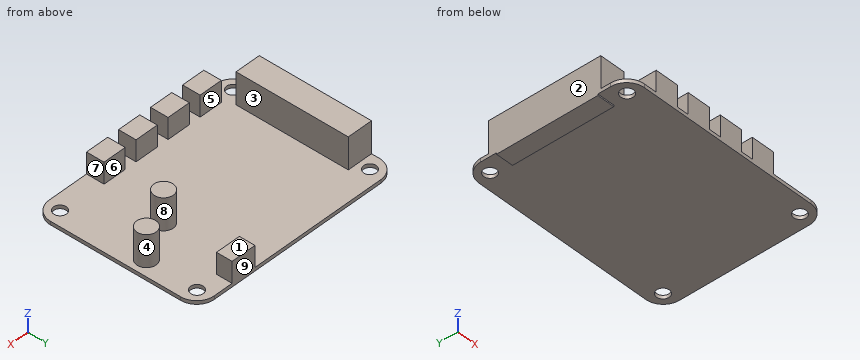
```python
from build123d import *

# Parameters (mm, degrees)
SKETCH_2_R      = 1.8
EXTRUDE_1_DEPTH = 1
SKETCH_4_W      = 7.237291628
SKETCH_4_H      = 31.958994792
EXTRUDE_2_DEPTH = 9
SKETCH_5_W      = 6.609648953
SKETCH_5_H      = 4.992409467
SKETCH_5_W_2    = 7.131463344
SKETCH_5_H_2    = 4.436954379
EXTRUDE_3_DEPTH = 6
SKETCH_6_R      = 2.75
EXTRUDE_4_DEPTH = 9
SKETCH_7_W      = 5
SKETCH_7_H      = 28.854406725
EXTRUDE_5_DEPTH = 0.4


with BuildPart() as part:
    # 草图2 → 凸台-拉伸1 (new body)
    with BuildSketch(Plane.XY):
        with BuildLine():
            Line((-26, 23.5), (26, 23.5))
            ThreePointArc((26, 23.5), (29.535533906, 22.035533906), (31, 18.5))
            Line((31, 18.5), (31, -18.5))
            ThreePointArc((31, -18.5), (29.535533906, -22.035533906), (26, -23.5))
            Line((26, -23.5), (-26, -23.5))
            ThreePointArc((-26, -23.5), (-29.535533906, -22.035533906), (-31, -18.5))
            Line((-31, -18.5), (-31, 18.5))
            ThreePointArc((-31, 18.5), (-29.535533906, 22.035533906), (-26, 23.5))
        make_face()
        with Locations((27, 19.5)):
            Circle(SKETCH_2_R, mode=Mode.SUBTRACT)
        with Locations(Location((-27, 19.5, 0), (0, 0, 180))):
            Circle(SKETCH_2_R, mode=Mode.SUBTRACT)
        with Locations(Location((27, -19.5, 0), (0, 0, 180))):
            Circle(SKETCH_2_R, mode=Mode.SUBTRACT)
        with Locations((-27, -19.5)):
            Circle(SKETCH_2_R, mode=Mode.SUBTRACT)
    extrude(amount=EXTRUDE_1_DEPTH)

    # 草图4 → 凸台-拉伸2 (add)
    with BuildSketch(Plane.XY.offset(1)):
        with Locations((-27.381354186, 0.304371379)):
            Rectangle(SKETCH_4_W, SKETCH_4_H)
    extrude(amount=EXTRUDE_2_DEPTH)

    # 草图5 → 凸台-拉伸3 (add)
    with BuildSketch(Plane.XY.offset(1)):
        with Locations((-18.965120236, -21.003795266)):
            Rectangle(SKETCH_5_W, SKETCH_5_H)
        with Locations((-8.96367774, -21.003795266)):
            Rectangle(SKETCH_5_W, SKETCH_5_H)
        with Locations((1.037764754, -21.003795266)):
            Rectangle(SKETCH_5_W, SKETCH_5_H)
        with Locations((11.039207249, -21.003795266)):
            Rectangle(SKETCH_5_W, SKETCH_5_H)
        with Locations((16.866134615, 21.281522811)):
            Rectangle(SKETCH_5_W_2, SKETCH_5_H_2)
    extrude(amount=EXTRUDE_3_DEPTH)

    # 草图6 → 凸台-拉伸4 (add)
    with BuildSketch(Plane.XY.offset(1)):
        with Locations((26.719458911, 4.848201251)):
            Circle(SKETCH_6_R)
        with Locations((15.293444682, -0.687190124)):
            Circle(SKETCH_6_R)
    extrude(amount=EXTRUDE_4_DEPTH)

    # 草图7 → 凸台-拉伸5 (add)
    with BuildSketch(Plane(origin=(0, 0, 0), x_dir=(-1, 0, 0), z_dir=(0, 0, -1))):
        with Locations((28.5, -0.417423606)):
            Rectangle(SKETCH_7_W, SKETCH_7_H)
    extrude(amount=EXTRUDE_5_DEPTH)


solid = part.part
```
Input: part model. Units: mm. Frame: model coordinates. Face numbers are marked on the shaded views. A direction names the side the tool comes from. Give positions to 0.01 mm unless a question says otherwise; leave off trailing zeros. Write each loop counter-clockwise with the first axis right and the second up, starting at its lowest first coordinate (ties: lowest second). Pieces come first, ordered by that corner, then holes. Notation, with made-up numbers: (-28.75, 62) - (-9.75, 62) arc R19 cw to (-9.75, 82) - close; hole circle Ø11 at (43.25, -31). An arc over 180 degrees is marked (long way). Write item = value, one per line. Start each with the question number.
1) Cut plane D-D (x = -27). Return loops of the section in (y, z), and give its area (3 significant figures).
2) Material intervals for L1, parallel to X at y = -21.5, z = 6.5; L2, parallel to Y at x = -27, z = 0.7; L3, parallel to Y at x = 14, z = 2.5, sorted ascending. Write a range as [from, to].
3) Reachability of the marked faces 5, 6, 7, 8 and 9 from +Z, -Z, +X, -X, +Y, -Y: full face, straight path, thin tool, end or side. Return the list, or none.
4) Cut plane C-C (z = 2). Return loops of the section in (x, y), and give its area (3 significant figures).
5) Cut plane A-A (x = -18.5). Return loops of the section in (y, z), and give its area (3 significant figures).
6) Pin query (flat end, axial travel): pin 1 (5 mm diameter, centred on x = -10.5, z = 4, fed in from +Y); pin 2 (3 mm diameter, centred on x = 27, y = 19.5, fed in from +Z); pin 3 (1 mm diameter, centred on x = -8, y = 12.5, fed in from -Z); pin 4 (1.8 mm diameter, centred on x = 18, z = 3, fed in from -Y). Return the tip coordinate at first contact, or that it passes through.
7) Cut plane B-B (y = -19.5). Return loops of the section in (x, z), and give its area (3 significant figures).
8) Draft query along X for the marked faces 1, 2, 3 and 4. Return one class per face: pulls with the +X half, pulls with the -X half, needs draft (parallel to the pull), parting line crosses it, or undercut.
Answers follow:
q1.outline = (-23.4, 0) - (-21.3, 0) - (-21.3, 1) - (-23.4, 1) - close; (-17.7, 0) - (-14.84, 0) - (-14.84, -0.4) - (14.01, -0.4) - (14.01, 0) - (17.7, 0) - (17.7, 1) - (16.28, 1) - (16.28, 10) - (-15.68, 10) - (-15.68, 1) - (-17.7, 1) - close; (21.3, 0) - (23.4, 0) - (23.4, 1) - (21.3, 1) - close
q1.area = 339 mm^2
q2.L1 = [-22.27, -15.66], [-12.27, -5.66], [-2.27, 4.34], [7.73, 14.34]
q2.L2 = [-23.4, -21.3], [-17.7, 17.7], [21.3, 23.4]
q2.L3 = [-23.5, -18.51], [-3.11, 1.74], [19.06, 23.5]
q3.face_5 = +Z, +X, -X, +Y
q3.face_6 = +Z, +X, -X
q3.face_7 = +Z, +X, -Y
q3.face_8 = +Z
q3.face_9 = +Z, -Z, +X, -X, +Y
q4.outline = (-31, -15.68) - (-23.76, -15.68) - (-23.76, 16.28) - (-31, 16.28) - close; (-22.27, -23.5) - (-15.66, -23.5) - (-15.66, -18.51) - (-22.27, -18.51) - close; (-12.27, -23.5) - (-5.66, -23.5) - (-5.66, -18.51) - (-12.27, -18.51) - close; (-2.27, -23.5) - (4.34, -23.5) - (4.34, -18.51) - (-2.27, -18.51) - close; (7.73, -23.5) - (14.34, -23.5) - (14.34, -18.51) - (7.73, -18.51) - close; circle Ø5.5 at (15.29, -0.69); (13.3, 19.06) - (20.43, 19.06) - (20.43, 23.5) - (13.3, 23.5) - close; circle Ø5.5 at (26.72, 4.85)
q4.area = 442 mm^2
q5.outline = (-23.5, 0) - (23.5, 0) - (23.5, 1) - (-18.51, 1) - (-18.51, 7) - (-23.5, 7) - close
q5.area = 77.0 mm^2
q6.pin_1 = -18.51
q6.pin_2 = through
q6.pin_3 = 0
q6.pin_4 = -2.76
q7.outline = (-30.9, 0) - (-28.8, 0) - (-28.8, 1) - (-30.9, 1) - close; (-25.2, 0) - (25.2, 0) - (25.2, 1) - (14.34, 1) - (14.34, 7) - (7.73, 7) - (7.73, 1) - (4.34, 1) - (4.34, 7) - (-2.27, 7) - (-2.27, 1) - (-5.66, 1) - (-5.66, 7) - (-12.27, 7) - (-12.27, 1) - (-15.66, 1) - (-15.66, 7) - (-22.27, 7) - (-22.27, 1) - (-25.2, 1) - close; (28.8, 0) - (30.9, 0) - (30.9, 1) - (28.8, 1) - close
q7.area = 213 mm^2
q8.face_1 = needs draft
q8.face_2 = pulls with the -X half
q8.face_3 = undercut
q8.face_4 = undercut
